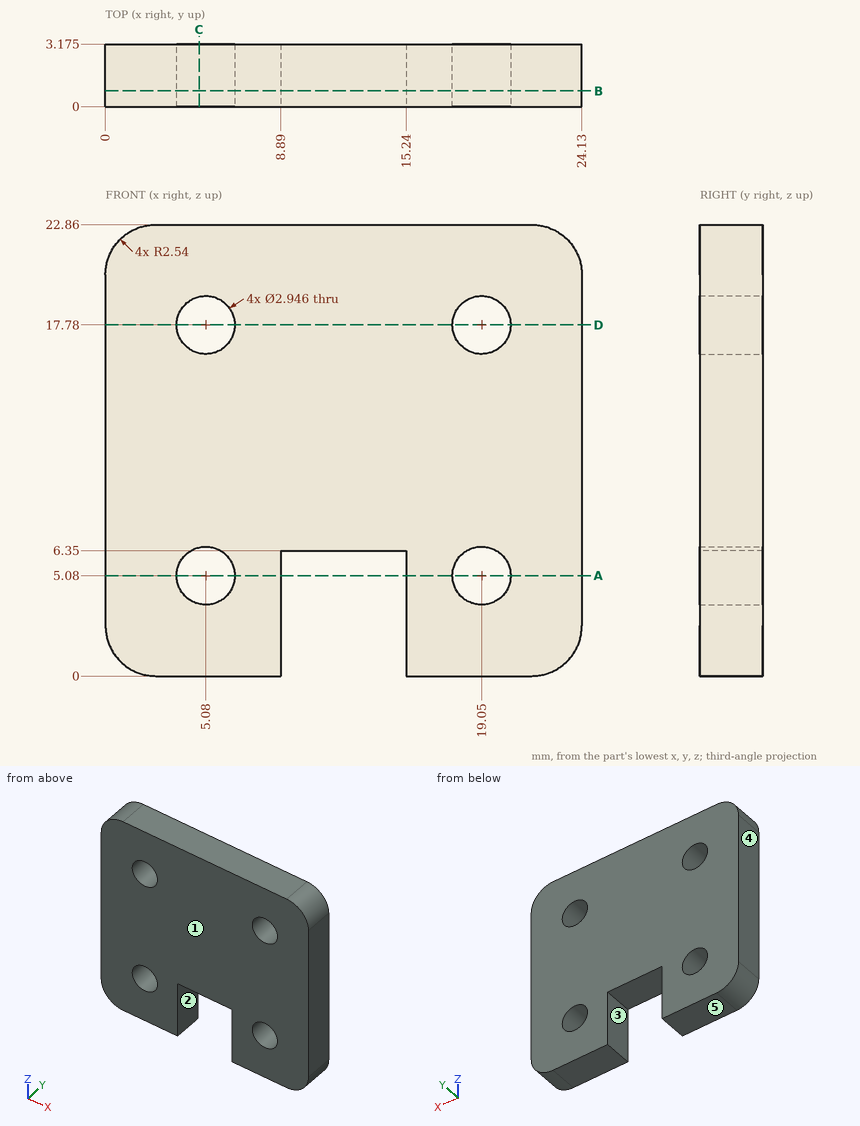
Geometry check sheet. Reference: drawing and pictorial views, mm from the part's lowest x, y, z. A direction names the side the tool comes from. Give positions to 0.01 mm unless a question says otherwise; leave off trailing zeros. Loops run counter-clockwise (first coordinate to the right, second up) from the corner with the lowest first, then second, coordinate; pieces in that order, holes last. Notation, with made-up numbers: M 22,12 L 44,12 A22 ccw 44,49 Z; hole C 21,83 d8. An arc over 180 degrees is marked long. Use a Markdown table: item, result. Add a question column.
Q1. Sectioned sample at B-B, the plane y = 0.8. Record the cut outline in (x, z).
Q2. Scan lines: line 1 along Z through (x, y) = (5.08, 0.7); line 2 along X through (y, z) = (1.35, 17.78); line 3 along Z through (x, y) = (5.5, 1.15). Record each from-to range of solid material in increasing order. Write a range as [from, to].
Q3. Sectioned sample at D-D, the plane z = 17.78. Record the cut outline in (x, y) (1 decimal).
Q4. Mould release check, pull along X, two halves, no side actions. Record for the marked faces 3, 4 and 5: pulls with the +X half, pulls with the -X half, needs draft (parallel to the pull), parting line crosses it, or undercut.
Q5. Sectioned sample at A-A, the plane z = 5.08. Record the cut outline in (x, y) (1 decimal).
Q6. Sectioned sample at C-C, the plane x = 4.75. Record the cut outline in (y, z) (1 decimal).
Q7. Go/stop test with flat-tipped pins: pin 1 (4 mm diameter, centred on x = 5.08, z = 17.78, fed in from +Y) (3 decimals); pin 2 (1.6 mm diameter, centred on x = 12.5, y = 1.5, fed in from -Z). Record where each tip stops, or that it passes through.
Q8. Tool access check on the marked faces 1 and 2. Record the directions out of +Z, -Z, +X, -X, +Y, -Y that give a thin tool (end or side, any length) a straight path to the whole face; none if there is none.
Verdict:
| question | item | result |
|---|---|---|
| 1 | outline | M 0,2.54 A2.54 ccw 2.54,0 L 8.89,0 L 8.89,6.35 L 15.24,6.35 L 15.24,0 L 21.59,0 A2.54 ccw 24.13,2.54 L 24.13,20.32 A2.54 ccw 21.59,22.86 L 2.54,22.86 A2.54 ccw 0,20.32 Z; hole C 5.08,5.08 d2.95; hole C 5.08,17.78 d2.95; hole C 19.05,5.08 d2.95; hole C 19.05,17.78 d2.95 |
| 2 | line 1 | [0, 3.61], [6.55, 16.31], [19.25, 22.86] |
| 2 | line 2 | [0, 3.61], [6.55, 17.58], [20.52, 24.13] |
| 2 | line 3 | [0, 3.67], [6.49, 16.37], [19.19, 22.86] |
| 3 | outline | M 0,0 L 3.6,0 L 3.6,3.2 L 0,3.2 Z; M 6.6,0 L 17.6,0 L 17.6,3.2 L 6.6,3.2 Z; M 20.5,0 L 24.1,0 L 24.1,3.2 L 20.5,3.2 Z |
| 4 | face 3 | undercut |
| 4 | face 4 | pulls with the -X half |
| 4 | face 5 | needs draft |
| 5 | outline | M 0,0 L 3.6,0 L 3.6,3.2 L 0,3.2 Z; M 6.6,0 L 8.9,0 L 8.9,3.2 L 6.6,3.2 Z; M 15.2,0 L 17.6,0 L 17.6,3.2 L 15.2,3.2 Z; M 20.5,0 L 24.1,0 L 24.1,3.2 L 20.5,3.2 Z |
| 6 | outline | M 0,0 L 3.2,0 L 3.2,3.6 L 0,3.6 Z; M 0,6.5 L 3.2,6.5 L 3.2,16.3 L 0,16.3 Z; M 0,19.2 L 3.2,19.2 L 3.2,22.9 L 0,22.9 Z |
| 7 | pin 1 | y = 3.175 |
| 7 | pin 2 | z = 6.35 |
| 8 | face 1 | +Z, -Z, +X, -X, -Y |
| 8 | face 2 | -Z, +Y, -Y |
